Source: CAD feature listing. Evaluate the final solid. Frame: model axes, mm. Coordinates: 2 decimals unless noted, no trailing zeros. Write each loop counter-clockwise with the first axis right and the second up, starting at its lowest first coordinate (ties: lowest second). Pieces come first, ordered by that corner, then holes. Notation, with made-up numbers: M 30,32.25 L 63,32.25 A11 ccw 63,40.25 Z; hole C 11,20 d8. An arc over 180 degrees is marked long. Write item = value, one per line. Start each with the question number.
1. Section query C-C (x = -23.5). Output: boundary loops of the cut face in (y, z) (3 decimals).
2. Pin query (flat end, axial travel): pin 1 Ø4 at (x, y) = (0, 114.3) entering from +Z. Return the tip coordinate at first contact, or that it passes through.
3. Line query: line 1 along Y through (x, z) = (-44.45, 1.6) (3 decimals); line 2 along Y through (x, z) = (-45.5, 1.6); line 3 along X through (y, z) = (114, 1.45). Output: solid intervals per line, ascending.
4. Section query A-A (y = 113). Output: boundary loops of the cut face in (x, z) (3 decimals).
5. Section query D-D (y = 78.5). Output: boundary loops of the cut face in (x, z) (3 decimals), then the cut area to 3 significant figures.
6. Section query B-B (z = 1.1). Give the number of separate pieces and of enclosed holes in the cut face, then the cut area to 3 significant figures.
```python
from build123d import *

# Parameters (mm, degrees)
F0_R     = 3.175
F1_DEPTH = 3.175


with BuildPart() as f1:
    # F0 (on Top) → F1 (new body)
    with BuildSketch(Plane.XY):
        with BuildLine():
            ThreePointArc((9.481007, -0.9144), (9.513995, -0.457729), (9.525, 0))
            ThreePointArc((9.525, 0), (6.613827, 6.854408), (-0.340179, 9.518923))
            ThreePointArc((-0.340179, 9.518923), (-9.525, 0), (-0.340179, -9.518923))
            ThreePointArc((-0.340179, -9.518923), (6.276794, -7.16432), (9.481007, -0.9144))
        make_face()
        Circle(F0_R, mode=Mode.SUBTRACT)
        with BuildLine():
            ThreePointArc((-0.340179, 9.518923), (6.613827, 6.854408), (9.525, 0))
            ThreePointArc((9.525, 0), (9.513995, -0.457729), (9.481007, -0.9144))
            Line((9.481007, -0.9144), (15.548852, 62.000384))
            ThreePointArc((15.548852, 62.000384), (0, 47.879), (-15.548852, 62.000384))
            Line((-15.548852, 62.000384), (-11.287798, 17.819412))
            ThreePointArc((-11.287798, 17.819412), (-13.280149, 11.634986), (-19.148911, 8.846754))
            Line((-19.148911, 8.846754), (-44.733482, 7.932436))
            ThreePointArc((-44.733482, 7.932436), (-38.938477, 5.712007), (-36.5125, 0))
            ThreePointArc((-36.5125, 0), (-38.938477, -5.712007), (-44.733482, -7.932436))
            Line((-44.733482, -7.932436), (-0.340179, -9.518923))
            ThreePointArc((-0.340179, -9.518923), (-9.525, 0), (-0.340179, 9.518923))
        make_face()
        with BuildLine():
            ThreePointArc((-15.548852, 62.000384), (0, 47.879), (15.548852, 62.000384))
            ThreePointArc((15.548852, 62.000384), (15.602953, 62.749325), (15.621, 63.5))
            ThreePointArc((15.621, 63.5), (15.592755, 64.438958), (15.508121, 65.37452))
            ThreePointArc((15.508121, 65.37452), (0, 79.121), (-15.508121, 65.37452))
            ThreePointArc((-15.508121, 65.37452), (-15.619862, 63.688555), (-15.548852, 62.000384))
        make_face()
        with Locations((0, 63.5)):
            Circle(F0_R, mode=Mode.SUBTRACT)
        with BuildLine():
            ThreePointArc((-44.733482, 7.932436), (-52.3875, 0), (-44.733482, -7.932436))
            ThreePointArc((-44.733482, -7.932436), (-38.938477, -5.712007), (-36.5125, 0))
            ThreePointArc((-36.5125, 0), (-38.938477, 5.712007), (-44.733482, 7.932436))
        make_face()
        with Locations((-44.45, 0)):
            Circle(F0_R, mode=Mode.SUBTRACT)
        with BuildLine():
            ThreePointArc((-15.508121, 65.37452), (0, 79.121), (15.508121, 65.37452))
            Line((15.508121, 65.37452), (9.456171, 115.443))
            ThreePointArc((9.456171, 115.443), (9.507777, 114.872535), (9.525, 114.3))
            ThreePointArc((9.525, 114.3), (-0.572535, 104.792223), (-9.456171, 115.443))
            Line((-9.456171, 115.443), (-15.508121, 65.37452))
        make_face()
        with Locations((3.175, 100.0125)):
            Circle(F0_R, mode=Mode.SUBTRACT)
        with BuildLine():
            ThreePointArc((9.525, 114.3), (9.507777, 114.872535), (9.456171, 115.443))
            ThreePointArc((9.456171, 115.443), (0, 123.825), (-9.456171, 115.443))
            ThreePointArc((-9.456171, 115.443), (-0.572535, 104.792223), (9.525, 114.3))
        make_face()
        with Locations((0, 114.3)):
            Circle(F0_R, mode=Mode.SUBTRACT)
    extrude(amount=F1_DEPTH)


solid = f1.part
```
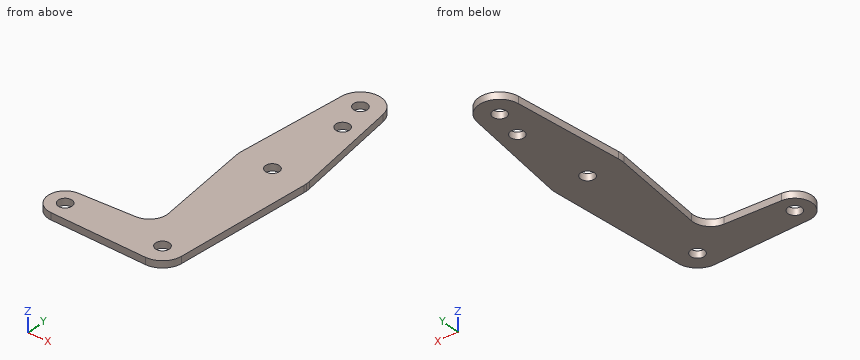
Results are:
q1.outline = M -8.691,0 L 8.691,0 L 8.691,3.175 L -8.691,3.175 Z
q2.pin_1 = through
q3.line_1 = -7.943 to -3.175, 3.175 to 7.943
q3.line_2 = -7.87 to -3, 3 to 7.87
q3.line_3 = -9.63 to -3.16, 3.16 to 9.63
q4.outline = M -9.751,0 L -2.897,0 L -2.897,3.175 L -9.751,3.175 Z; M 2.897,0 L 9.751,0 L 9.751,3.175 L 2.897,3.175 Z
q5.outline = M -13.922,0 L 13.922,0 L 13.922,3.175 L -13.922,3.175 Z
q5.area = 88.4 mm^2
q6.separate_pieces = 1
q6.enclosed_holes = 5
q6.area = 3,740 mm^2
